from build123d import *

# Parameters (mm, degrees)
BOSS_EXTRUDE1_DEPTH = 25
SKETCH2_W           = 40
SKETCH2_H           = 20
CUT_EXTRUDE1_DEPTH  = 20
FILLET1_R           = 10
FILLET2_R           = 10


with BuildPart() as part:
    # Sketch1 → Boss-Extrude1 (new, symmetric)
    with BuildSketch(Plane.XY):
        Polygon((0, 45), (-40, 45), (-40, 15), (-11.336760925, -45), (0, -45), align=None)
    extrude(amount=BOSS_EXTRUDE1_DEPTH, both=True)

    # Sketch2 → Cut-Extrude1 (cut)
    with BuildSketch(Plane(origin=(0, 45, 0), x_dir=(1, 0, 0), z_dir=(0, 1, 0))):
        with Locations((-20, 0)):
            Rectangle(SKETCH2_W, SKETCH2_H)
    extrude(amount=-CUT_EXTRUDE1_DEPTH, mode=Mode.SUBTRACT)

    # Fillet1
    fillet1_edges = [part.edges().sort_by_distance(p)[0] for p in [
        (-40, 45, -17.5),
        (-40, 45, 17.5),
    ]]
    fillet(fillet1_edges, radius=FILLET1_R)

    # Fillet2
    fillet2_edges = [part.edges().sort_by_distance(p)[0] for p in [
        (-11.336760925, -45, 0),
        (-40, 15, 0),
    ]]
    fillet(fillet2_edges, radius=FILLET2_R)


solid = part.part
Source: CAD feature listing. Evaluate the final solid. Frame: model axes, mm. A direction names the side the tool comes from. Round coordinates to 2 decimals unless told otherwise and drop trailing zeros. Order: outer loops, then holes, each group sorted by start corner. A loop starts at its lowest first (then second) coordinate and runs counter-clockwise, first axis right, second up. Notation, with made-up numbers: (26, 72.25) - (77, 72.25) arc R25 ccw to (77, 105.25) - close; hole circle Ø9 at (-25, 29). An arc over 180 degrees is marked (long way). Use a Markdown table: item, result. Add a question column.
1. Section query B-B (z = 9). Return the cut outline in (x, y), then the cut area to 3 significant figures.
2. Section query C-C (y = 39). Return the cut outline in (x, z).
3. Line query: probe 1 along Z at (x, y) = (-25.5, 27); probe 2 along Y at (x, z) = (-2, -6); probe 3 along Y at (x, z) = (-7.5, -13). Output: solid intervals per line, ascending.
4. Set-up query: faces 4 (the flat face through (-40, 24, 0)), 5 (the flat face through (-20, 35, 10)). Return all of +Z, -Z, +X, -X, +Y, -Y with unobstructed straight access to the full face (end or side cutting, diameter ignored); none if empty.
5. Mould query, pull axis Z, two halves, no side actions, for faces 1 (the flat face through (-20, 35, -10)), 2 (the flat face through (-16, 11, 25)), 3 (the flat face through (0, -1, 0)). Classes: +Z half, -Z half, draft (parallel to the pull), parting line (faces both ways), or undercut.
6. Section query A-A (x = -3). Return the cut outline in (y, z).
7. First-contact query: pin 1 (3 mm diameter, centred on x = -7, z = -14, fed in from -Y); pin 2 (6 mm diameter, centred on x = -24, z = -2.5, fed in from -Y); pin 3 (10 mm diameter, centred on x = -22.5, z = 3, fed in from +Y). Flat tips, straight axial feed; report the tip coordinate or a pass-through.
8. Section query D-D (z = 14). Return the cut outline in (x, y).
Derived:
| question | item | result |
|---|---|---|
| 1 | outline | (-40, 17.27) arc R10 ccw to (-39.02, 12.96) - (-14.05, -39.31) arc R10 ccw to (-5.03, -45) - (0, -45) - (0, 25) - (-40, 25) - close |
| 1 | area | 1,930 mm2 |
| 2 | outline | (-39.17, -25) - (0, -25) - (0, -10) - (-39.17, -10) - close; (-39.17, 10) - (0, 10) - (0, 25) - (-39.17, 25) - close |
| 3 | probe 1 | -25 to -10, 10 to 25 |
| 3 | probe 2 | -45 to 25 |
| 3 | probe 3 | -44.69 to 45 |
| 4 | face 4 | +Z, -Z, -X, +Y, -Y |
| 4 | face 5 | +X, -X, +Y |
| 5 | face 1 | undercut |
| 5 | face 2 | +Z half |
| 5 | face 3 | draft |
| 6 | outline | (-45, -25) - (45, -25) - (45, -10) - (25, -10) - (25, 10) - (45, 10) - (45, 25) - (-45, 25) - close |
| 7 | pin 1 | y = -44.99 |
| 7 | pin 2 | y = -24.77 |
| 7 | pin 3 | y = 25 |
| 8 | outline | (-40, 17.27) arc R10 ccw to (-39.02, 12.96) - (-14.05, -39.31) arc R10 ccw to (-5.03, -45) - (0, -45) - (0, 45) - (-30, 45) arc R10 ccw to (-40, 35) - close |
